from build123d import *

# Parameters (mm, degrees)
REDONDEO1_R = 0.5


with BuildPart() as part:
    # Croquis1 → Revolución1 (revolve)
    with BuildSketch(Plane.XY, mode=Mode.PRIVATE) as revoluci_n1_sk:
        Polygon((-8, 1.873006462), (-8, 3.730556499), (-8.240342635, 4.120291582), (-8.240342635, 4.539307424), (-9.558967924, 4.539307424), (-9.999624488, 4.02630535), (-9.999624488, 1.503449512), (-8.897118424, 1.503449512), (-8.250134341, 0.475546819), (-8, 0.475546819), (-8, 0.749389269), (-8.474621749, 1.503449512), align=None)
    revolve(revoluci_n1_sk.sketch.rotate(Axis((0, 26.098695966, 0), (0, -1, 0)), 270), axis=Axis((0, 26.098695966, 0), (0, -1, 0)))

    # Redondeo1
    redondeo1_edges = [part.edges().sort_by_distance(p)[0] for p in [
        (0, 1.503449512, -8.897118424),
    ]]
    fillet(redondeo1_edges, radius=REDONDEO1_R)


solid = part.part
The model under review builds one solid part; all positions refer to its coordinate system, in mm. A direction names the side the tool comes from. Give positions to 0.01 mm unless a question says otherwise; leave off trailing zeros. Write each loop counter-clockwise with the first axis right and the second up, starting at its lowest first coordinate (ties: lowest second). Pieces come first, ordered by that corner, then holes.
1. Add section B-B, the plane x = 0. Write out the cut boundary in (y, z), plus the area to 3 significant figures.
2. Add section C-C, the plane y = 2.7. Write out the cut boundary in (x, z), plus the area to 3 significant figures.
3. Add section A-A, the plane z = 0. Write out the cut boundary in (x, y), plus the area to 3 significant figures.
4. Draft analysis for pull direction X (two halves, no side actions). For faces 3 (the cylindrical face through (7.81, 2.81, -1.73)), 4 (the cylindrical face through (6, 3, -8)), 5 (the flat face through (-8, 4.539, -3)), state which applies: +X half, -X half, draft (parallel to the pull), parting line (faces both ways), or undercut.
5. Wall thickness on L1, parallel to X at y = 2.9, z = 0; L2, parallel to X at y = 1.35, z = -0.5; L3, parallel to Y at x = -8, z = 4.5: over which ranges is each line inside the solid? List them lowest first.
6. Tool access review of faces 1 (the flat face through (9, 1.503, 3)), 2 (the cylindrical face through (-2.48, 4.33, 7.86)): name each direction out of +Z, -Z, +X, -X, +Y, -Y from which nothing blocks a thin tool from reaching the whole face with its end or side.
7. For P1, Ø3, axis at x = -2, z = -5, coming from the +Y side; P2, Ø1.5, axis at y = 3, z = -3.5, coming from the -X side, all flat-tipped, find the tip position at first contact; note any pin that passes through.
Worked answers:
1. outline: (0.48, -8.25) - (1.27, -8.75) arc R0.5 cw to (1.5, -9.17) - (1.5, -10) - (4.03, -10) - (4.54, -9.56) - (4.54, -8.24) - (4.12, -8.24) - (3.73, -8) - (1.87, -8) - (1.5, -8.47) - (0.75, -8) - (0.48, -8) - close; (0.48, 8) - (0.75, 8) - (1.5, 8.47) - (1.87, 8) - (3.73, 8) - (4.12, 8.24) - (4.54, 8.24) - (4.54, 9.56) - (4.03, 10) - (1.5, 10) - (1.5, 9.17) arc R0.5 cw to (1.27, 8.75) - (0.48, 8.25) - close
1. area: 12.3 mm2
2. outline: circle Ø20 at (0, 0); hole circle Ø16 at (0, 0)
2. area: 113 mm2
3. outline: (-10, 1.5) - (-9.17, 1.5) arc R0.5 cw to (-8.75, 1.27) - (-8.25, 0.48) - (-8, 0.48) - (-8, 0.75) - (-8.47, 1.5) - (-8, 1.87) - (-8, 3.73) - (-8.24, 4.12) - (-8.24, 4.54) - (-9.56, 4.54) - (-10, 4.03) - close; (8, 0.48) - (8.25, 0.48) - (8.75, 1.27) arc R0.5 cw to (9.17, 1.5) - (10, 1.5) - (10, 4.03) - (9.56, 4.54) - (8.24, 4.54) - (8.24, 4.12) - (8, 3.73) - (8, 1.87) - (8.47, 1.5) - (8, 0.75) - close
3. area: 12.3 mm2
4. face 3: undercut
4. face 4: parting line
4. face 5: draft
5. L1: x = -10 to -8, 8 to 10
5. L2: x = -8.8 to -8.36, 8.36 to 8.8
5. L3: y = 1.5 to 4.54
6. face 1: -Y
6. face 2: +Y
7. P1: passes through
7. P2: stops at x = -9.61
